Geometry: see drawing. Coordinates: mm, zero at the bounding-box minimum. A direction names the side the tool comes from. Round coordinates to 2 decimals unless told otherwise and drop trailing zeros. Write each loop counter-clockwise with the first axis right and the second up, starting at its lowest first coordinate (ties: lowest second). Pieces come first, ordered by that corner, then holes.
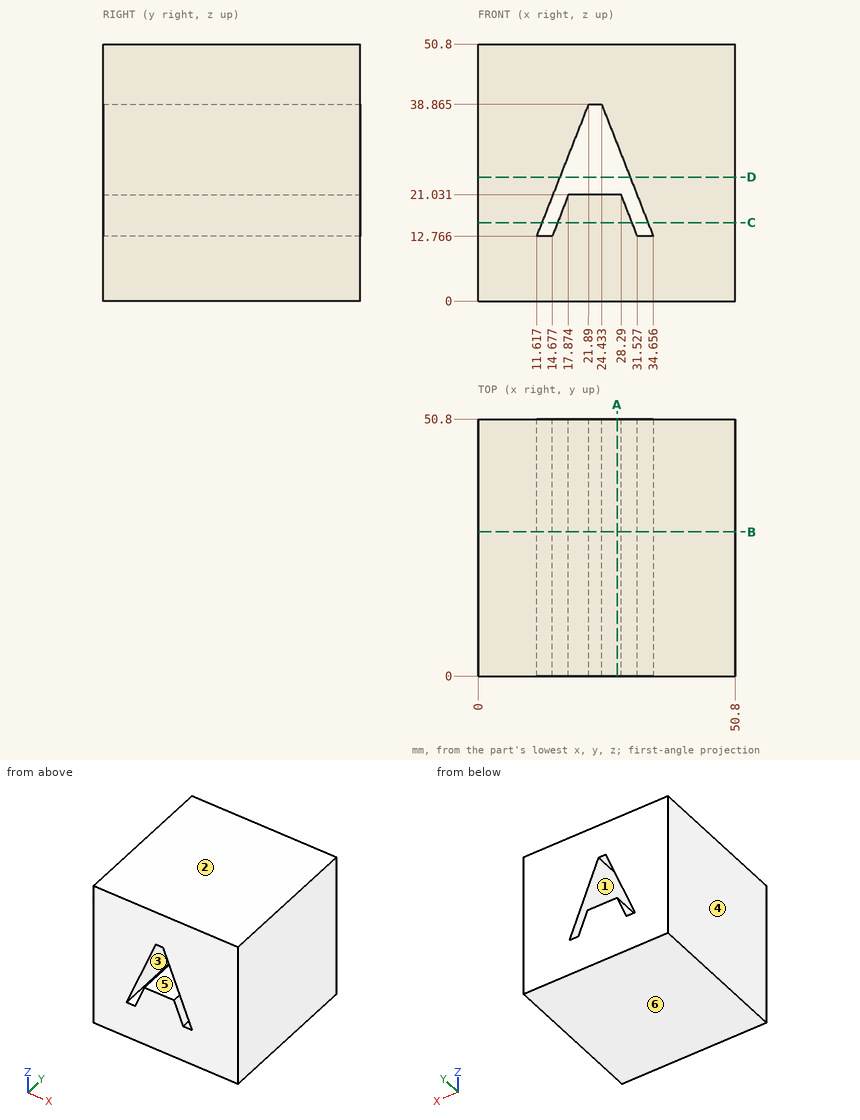
Q1. Line query: line 1 (X direction, y = 31.5, z = 20) (1 decimal); line 2 (X direction, y = 26, z = 23.5); line 3 (X direction, y = 24, z = 19.5). Output: solid intervals per line, ascending.
Q2. Section query C-C, the plane z = 15.5. Output: boundary loops of the cut face in (x, y) (1 decimal), and give its area (3 significant figures).
Q3. Set-up query: the marked faces 5 and 6. Return all of +Z, -Z, +X, -X, +Y, -Y with unobstructed straight access to the full face (end or side cutting, diameter ignored); none if empty.
Q4. Section query A-A, the plane x = 27.5. Output: boundary loops of the cut face in (y, z) (1 decimal), and give its area (3 significant figures).
Q5. Mould query, pull axis X, two halves, no side actions, for the marked faces 1, 2, 3 and 4. Classes: pulls with the +X half, pulls with the -X half, needs draft (parallel to the pull), parting line crosses it, or undercut.
Q6. Section query B-B, the plane y = 28.5. Output: boundary loops of the cut face in (x, z) (1 decimal), and give its area (3 significant figures).
Q7. Section query D-D, the plane z = 24.5. Output: boundary loops of the cut face in (x, y) (1 decimal).
Filled in:
1. line 1: x = 0 to 14.5, 17.5 to 28.7, 31.8 to 50.8
1. line 2: x = 0 to 15.84, 30.45 to 50.8
1. line 3: x = 0 to 14.27, 17.28 to 28.89, 32.02 to 50.8
2. outline: (0, 0) - (12.7, 0) - (12.7, 50.8) - (0, 50.8) - close; (15.7, 0) - (30.5, 0) - (30.5, 50.8) - (15.7, 50.8) - close; (33.6, 0) - (50.8, 0) - (50.8, 50.8) - (33.6, 50.8) - close
2. area: 2,270 mm2
3. face 5: +Y, -Y
3. face 6: -Z, +X, -X, +Y, -Y
4. outline: (0, 0) - (50.8, 0) - (50.8, 21) - (0, 21) - close; (0, 31) - (50.8, 31) - (50.8, 50.8) - (0, 50.8) - close
4. area: 2,070 mm2
5. face 1: undercut
5. face 2: needs draft
5. face 3: undercut
5. face 4: pulls with the -X half
6. outline: (0, 0) - (50.8, 0) - (50.8, 50.8) - (0, 50.8) - close; hole (11.6, 12.8) - (14.7, 12.8) - (17.9, 21) - (28.3, 21) - (31.5, 12.8) - (34.7, 12.8) - (24.4, 38.9) - (21.9, 38.9) - close
6. area: 2,360 mm2
7. outline: (0, 0) - (16.2, 0) - (16.2, 50.8) - (0, 50.8) - close; (30.1, 0) - (50.8, 0) - (50.8, 50.8) - (30.1, 50.8) - close
